Input: part model. Units: mm. Frame: model coordinates. Face numbers are marked on the shaded views. A direction names the side the tool comes from. Round coordinates to 2 decimals unless told otherwise and drop trailing zeros. Order: outer loops, then holes, each group sorted by start corner. A loop starts at its lowest first (then second) coordinate and runs counter-clockwise, first axis right, second up. Notation, with made-up numbers: (30, 17.25) -> (74, 17.25) arc R29 cw to (74, 39.25) -> close; hole circle Ø2 at (26, 82). An arc over 180 degrees is marked (long way). Use a Markdown table: item, result.
from build123d import *

# Parameters (mm, degrees)
SKETCH1_W                      = 50
SKETCH1_H                      = 50
BOSS_EXTRUDE1_DEPTH            = 19
SKETCH2_W                      = 44
SKETCH2_H                      = 44
CUT_EXTRUDE1_DEPTH             = 16
CBORE_FOR_M6_SHCS1_D           = 6
CBORE_FOR_M6_SHCS1_CBORE_D     = 11
CBORE_FOR_M6_SHCS1_CBORE_DEPTH = 1
SKETCH6_W                      = 38
SKETCH6_H                      = 12
CUT_EXTRUDE2_DEPTH             = 16
FILLET1_R                      = 1
FILLET3_R                      = 1
CUT_EXTRUDE3_DEPTH             = 51
CUT_EXTRUDE4_DEPTH             = 51
SKETCH9_W                      = 1
SKETCH9_H                      = 29.077623466
CUT_EXTRUDE5_DEPTH             = 10
SKETCH10_W                     = 28.99096046
SKETCH10_H                     = 1
CUT_EXTRUDE6_DEPTH             = 10
SKETCH11_W                     = 28.99096046
SKETCH11_H                     = 1
CUT_EXTRUDE7_DEPTH             = 10
SKETCH12_W                     = 1
SKETCH12_H                     = 29.077623466
CUT_EXTRUDE8_DEPTH             = 10


with BuildPart() as part:
    # Sketch1 → Boss-Extrude1 (new body)
    with BuildSketch(Plane(origin=(0, 0, 0), x_dir=(1, 0, 0), z_dir=(0, 1, 0))):
        Rectangle(SKETCH1_W, SKETCH1_H)
    extrude(amount=BOSS_EXTRUDE1_DEPTH)

    # Sketch2 → Cut-Extrude1 (cut)
    with BuildSketch(Plane(origin=(0, 19, 0), x_dir=(1, 0, 0), z_dir=(0, 1, 0))):
        Rectangle(SKETCH2_W, SKETCH2_H)
    extrude(amount=-CUT_EXTRUDE1_DEPTH, mode=Mode.SUBTRACT)

    # CBORE for M6 SHCS1 (through all)
    with Locations(Plane(origin=(-12.5, 3, 0), x_dir=(0, 0, 1), z_dir=(0, 1, 0))):
        with Locations((0, 0), (0, 25)):
            CounterBoreHole(CBORE_FOR_M6_SHCS1_D / 2, CBORE_FOR_M6_SHCS1_CBORE_D / 2, CBORE_FOR_M6_SHCS1_CBORE_DEPTH)

    # Sketch6 → Cut-Extrude2 (cut)
    with BuildSketch(Plane(origin=(0, 3, 0), x_dir=(1, 0, 0), z_dir=(0, 1, 0))):
        with Locations((0, -13)):
            Rectangle(SKETCH6_W, SKETCH6_H)
        with Locations((0, 13)):
            Rectangle(SKETCH6_W, SKETCH6_H)
    extrude(amount=-CUT_EXTRUDE2_DEPTH, mode=Mode.SUBTRACT)

    # Fillet1
    fillet1_edges = [part.edges().sort_by_distance(p)[0] for p in [
        (-22, 11, 22),
        (-22, 11, -22),
        (22, 11, -22),
        (22, 11, 22),
        (-19, 1.5, 19),
        (-19, 1.5, 7),
        (19, 1.5, 7),
        (19, 1.5, 19),
        (-19, 1.5, -7),
        (-19, 1.5, -19),
        (19, 1.5, -19),
        (19, 1.5, -7),
    ]]
    fillet(fillet1_edges, radius=FILLET1_R)

    # Fillet3
    fillet3_edges = [part.edges().sort_by_distance(p)[0] for p in [
        (-25, 9.5, -25),
        (25, 9.5, -25),
        (25, 9.5, 25),
        (-25, 9.5, 25),
    ]]
    fillet(fillet3_edges, radius=FILLET3_R)

    # Sketch7 → Cut-Extrude3 (cut, through all)
    with BuildSketch(Plane(origin=(25, 0, 0), x_dir=(0, 0, -1), z_dir=(1, 0, 0))):
        Polygon((14.538811733, 5.5), (-14.538811733, 5.5), (-18, 19), (18, 19), align=None)
    extrude(amount=-CUT_EXTRUDE3_DEPTH, mode=Mode.SUBTRACT)

    # Sketch8 → Cut-Extrude4 (cut, through all)
    with BuildSketch(Plane.XY.offset(25)):
        Polygon((-18, 19), (18, 19), (14.49548023, 5.330990042), (-14.49548023, 5.330990042), align=None)
    extrude(amount=-CUT_EXTRUDE4_DEPTH, mode=Mode.SUBTRACT)

    # Sketch9 → Cut-Extrude5 (cut)
    with BuildSketch(Plane(origin=(0, 5.5, 0), x_dir=(1, 0, 0), z_dir=(0, 1, 0))):
        with Locations((24.5, 0)):
            Rectangle(SKETCH9_W, SKETCH9_H)
    extrude(amount=-CUT_EXTRUDE5_DEPTH, mode=Mode.SUBTRACT)

    # Sketch10 → Cut-Extrude6 (cut)
    with BuildSketch(Plane(origin=(0, 5.330990042, 0), x_dir=(1, 0, 0), z_dir=(0, 1, 0))):
        with Locations((0, -24.5)):
            Rectangle(SKETCH10_W, SKETCH10_H)
    extrude(amount=-CUT_EXTRUDE6_DEPTH, mode=Mode.SUBTRACT)

    # Sketch11 → Cut-Extrude7 (cut)
    with BuildSketch(Plane(origin=(0, 5.330990042, 0), x_dir=(1, 0, 0), z_dir=(0, 1, 0))):
        with Locations((0, 24.5)):
            Rectangle(SKETCH11_W, SKETCH11_H)
    extrude(amount=-CUT_EXTRUDE7_DEPTH, mode=Mode.SUBTRACT)

    # Sketch12 → Cut-Extrude8 (cut)
    with BuildSketch(Plane(origin=(0, 5.5, 0), x_dir=(1, 0, 0), z_dir=(0, 1, 0))):
        with Locations((-24.5, 0)):
            Rectangle(SKETCH12_W, SKETCH12_H)
    extrude(amount=-CUT_EXTRUDE8_DEPTH, mode=Mode.SUBTRACT)


solid = part.part
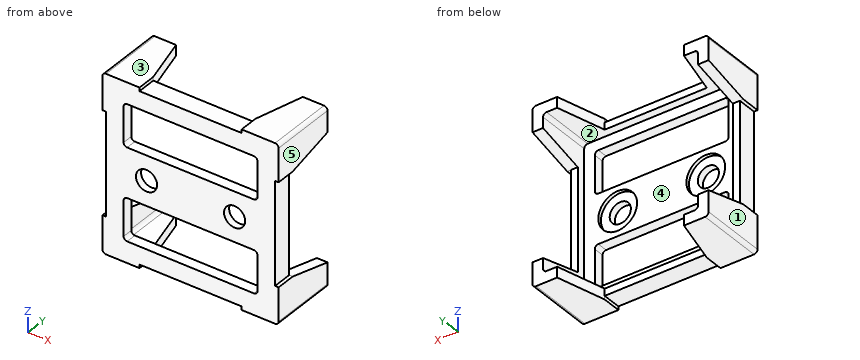
1) Draft query along Z for the marked faces 3, 4 and 5. Return one class per face: released by +Z, released by -Z, zero draft, split by the parting line, or undercut.
Answer key:
| item | result |
|---|---|
| face 3 | released by +Z |
| face 4 | undercut |
| face 5 | zero draft |
2) Contact query for flat-ended pins moving along their axis: P1, Ø3, axis at x = -0.5, y = 8.5, coming from the +Z side; P2, Ø13, axis at x = 3, z = -3, coming from the +Y side; P3, Ø3.5, axis at x = -6, y = 1.5, coming from the +Z side; P4, Ø6, axis at y = 3.5, z = 1, coming from the +X side. Output: stop coordinate, or through.
Answer key:
| item | result |
|---|---|
| P1 | passes through |
| P2 | stops at y = 3 |
| P3 | stops at z = 24 |
| P4 | stops at x = 24 |
3) Cut plane C-C on z = 0. Return loops of the section in (x, y).
Answer key:
| item | result |
|---|---|
| outline | (-24, 0) -> (-15.5, 0) -> (-15.5, 2) -> (-18, 2) -> (-18, 3) -> (-22, 3) -> (-22, 5.5) -> (-24, 5.5) -> close; (-9.5, 0) -> (9.5, 0) -> (9.5, 2) -> (7, 2) -> (7, 3) -> (-7, 3) -> (-7, 2) -> (-9.5, 2) -> close; (15.5, 0) -> (24, 0) -> (24, 5.5) -> (22, 5.5) -> (22, 3) -> (18, 3) -> (18, 2) -> (15.5, 2) -> close |
4) Cut plane A-A on x = -6. Return loops of the section in (y, z).
Answer key:
| item | result |
|---|---|
| outline | (0, -24) -> (5.33, -24) -> (5.33, -22) -> (3, -22) -> (3, -19) -> (0, -19) -> close; (0, -7) -> (3, -7) -> (3, 7) -> (0, 7) -> close; (0, 19) -> (3, 19) -> (3, 22) -> (5.33, 22) -> (5.33, 24) -> (0, 24) -> close |
5) Cut plane D-D on x = -12.5. Return loops of the section in (y, z).
Answer key:
| item | result |
|---|---|
| outline | (0, -24) -> (5.33, -24) -> (5.33, -22) -> (3, -22) -> (3, -19) -> (0, -19) -> close; (0, -7) -> (3, -7) -> (3, -5.5) -> (2, -5.5) -> (2, -3) -> (0, -3) -> close; (0, 3) -> (2, 3) -> (2, 5.5) -> (3, 5.5) -> (3, 7) -> (0, 7) -> close; (0, 19) -> (3, 19) -> (3, 22) -> (5.33, 22) -> (5.33, 24) -> (0, 24) -> close |
6) Set-up query: the marked faces 1 and 2. Return all of +Z, -Z, +X, -X, +Y, -Y with unobstructed straight access to the full face (end or side cutting, diameter ignored); none if empty.
Answer key:
| item | result |
|---|---|
| face 1 | +Z, -Z, -X, +Y, -Y |
| face 2 | +Y |
7) Cut plane B-B on y = 7.25. State how many separate pieces and enclosed holes the cut face has, and give its area (3 significant figures).
Answer key:
| item | result |
|---|---|
| separate pieces | 4 |
| enclosed holes | 0 |
| area | 204 mm^2 |
8) Ray query, probe 1 along X at (y, z) = (2.6, 0); probe 2 along X at (y, z) = (1, -16); probe 3 along Z at (x, y) = (18.5, 17). Return the intervals inside material, ascending.
Answer key:
| item | result |
|---|---|
| probe 1 | x = -24 to -18, -7 to 7, 18 to 24 |
| probe 2 | x = -25 to -19, 19 to 25 |
| probe 3 | z = -25 to -22, 22 to 25 |
